from build123d import *

# Parameters (mm, degrees)
SKETCH1_R           = 10
BOSS_EXTRUDE1_DEPTH = 10
SKETCH1_3_W         = 40
SKETCH1_3_H         = 10
BOSS_EXTRUDE2_DEPTH = 50
FILLET1_R           = 20
SKETCH2_R           = 10
CUT_EXTRUDE1_DEPTH  = 10


with BuildPart() as part:
    # Sketch1 → Boss-Extrude1 (new body)
    with BuildSketch(Plane(origin=(0, 0, 0), x_dir=(0, 0, -1), z_dir=(1, 0, 0))):
        with BuildLine():
            ThreePointArc((0, 20), (-20, 0), (0, -20))
            Line((0, -20), (40, -20))
            Line((40, -20), (40, -30))
            Line((40, -30), (70, -30))
            Line((70, -30), (70, -20))
            Line((70, -20), (30, 20))
            Line((30, 20), (0, 20))
        make_face()
        Circle(SKETCH1_R, mode=Mode.SUBTRACT)
    extrude(amount=BOSS_EXTRUDE1_DEPTH)

    # Sketch1<3> → Boss-Extrude2 (add)
    with BuildSketch(Plane(origin=(0, 0, 0), x_dir=(0, 0, -1), z_dir=(1, 0, 0))):
        with Locations((20, -25)):
            Rectangle(SKETCH1_3_W, SKETCH1_3_H)
    extrude(amount=BOSS_EXTRUDE2_DEPTH)

    # Fillet1
    fillet1_edges = [part.edges().sort_by_distance(p)[0] for p in [
        (50, -25, -40),
        (50, -25, 0),
    ]]
    fillet(fillet1_edges, radius=FILLET1_R - 0.0001)  # a hair under: the kernel refuses the full size

    # Sketch2 → Cut-Extrude1 (cut)
    with BuildSketch(Plane(origin=(0, -20, 0), x_dir=(1, 0, 0), z_dir=(0, 1, 0))):
        with Locations(Location((30, 20, 0), (0, 0, 270))):
            Circle(SKETCH2_R)
    extrude(amount=-CUT_EXTRUDE1_DEPTH, mode=Mode.SUBTRACT)


solid = part.part
The model under review builds one solid part; all positions refer to its coordinate system, in mm. A direction names the side the tool comes from. Give positions to 0.01 mm unless a question says otherwise; leave off trailing zeros. Order: outer loops, then holes, each group sorted by start corner. A loop starts at its lowest first (then second) coordinate and runs counter-clockwise, first axis right, second up. Notation, with made-up numbers: M -15.75,-32.5 L 8.25,-32.5 A34 cw 8.25,-0.5 Z; hole C -9,27 d4. An arc over 180 degrees is marked long. Answer in a Markdown table with one row per item. Add a question column.
1. Add section A-A on y = 0. State the section outline as (x, z) points, plus the area to 3 significant figures.
2. To check wall thickness, follow line 1 along X through (y, z) = (-26, -20); line 2 along X through (y, z) = (14, -17); line 3 along Y through (x, z) = (13.5, -8). State the ranges of each line that lie inside material, in increasing order.
3. Machinability: for faces 1 (the flat face through (20, -25, -40)), 2 (the flat face through (21, -20, -15)), 3 (the flat face through (15, -25, 0)), which of the approach directions +Z, -Z, +X, -X, +Y, -Y give a long, thin tool a straight path to every point of the face, cutting with its end or side? Answer none if there is none.
4. For pin 1 Ø3 at (y, z) = (14.5, 0) entering from -X; pin 2 Ø8 at (y, z) = (-5, -24) entering from +X; pin 3 Ø8 at (x, y) = (16.5, -23.5) entering from +Z; pin 4 Ø1 at (x, y) = (41.5, -22.5) entering from -Z, all flat-tipped, find the tip position at first contact; note any pin that passes through.
5. Add section D-D on z = -13. State the section outline as (x, y) points.
6. Add section B-B on z = 6. State the section outline as (x, y) points, plus the area to 3 significant figures.
7. Mouldability with a two-part tool opening along Y and no side actions: class faces 4 (the flat face through (5, 20, -15)), 5 (the cylindrical face through (4.93, -9.76, 2.17)), 6 (the flat face through (0, -5, -24)) as released by +Y, released by -Y, zero draft, split by the parting line, or undercut.
The answers:
| question | item | result |
|---|---|---|
| 1 | outline | M 0,-50 L 10,-50 L 10,-10 L 0,-10 Z; M 0,10 L 10,10 L 10,20 L 0,20 Z |
| 1 | area | 500 mm2 |
| 2 | line 1 | 0 to 20, 40 to 50 |
| 2 | line 2 | 0 to 10 |
| 2 | line 3 | -30 to -20 |
| 3 | face 1 | -Z, +X, +Y, -Y |
| 3 | face 2 | +Z, -Z, +X, +Y |
| 3 | face 3 | +Z, +X, -X, -Y |
| 4 | pin 1 | x = 0 |
| 4 | pin 2 | x = 10 |
| 4 | pin 3 | z = 0 |
| 4 | pin 4 | z = -36.7 |
| 5 | outline | M 0,-30 L 22.86,-30 L 22.86,-20 L 10,-20 L 10,20 L 0,20 Z; M 37.14,-30 L 48.74,-30 L 48.74,-20 L 37.14,-20 Z |
| 6 | outline | M 0,-19.08 L 10,-19.08 L 10,-8 L 0,-8 Z; M 0,8 L 10,8 L 10,19.08 L 0,19.08 Z |
| 6 | area | 222 mm2 |
| 7 | face 4 | released by +Y |
| 7 | face 5 | undercut |
| 7 | face 6 | zero draft |
